from build123d import *

# Parameters (mm, degrees)
SKETCH1_R           = 0.8875
BOSS_EXTRUDE1_DEPTH = 2.5


with BuildPart() as part:
    # Sketch1 → Boss-Extrude1 (new body)
    with BuildSketch(Plane.XY):
        with BuildLine():
            Line((-40, 6.25), (-7.806247498, 6.25))
            ThreePointArc((-7.806247498, 6.25), (10, 0), (-7.806247498, -6.25))
            Line((-7.806247498, -6.25), (-40, -6.25))
            ThreePointArc((-40, -6.25), (-46.25, 0), (-40, 6.25))
        make_face()
        Circle(SKETCH1_R, mode=Mode.SUBTRACT)
        with Locations((-40, 0)):
            Circle(SKETCH1_R, mode=Mode.SUBTRACT)
        with Locations((0, 7.1)):
            Circle(SKETCH1_R, mode=Mode.SUBTRACT)
        with Locations((0, -7.1)):
            Circle(SKETCH1_R, mode=Mode.SUBTRACT)
        with Locations((-38.938319925, -3.387526445)):
            Circle(SKETCH1_R, mode=Mode.SUBTRACT)
        with BuildLine():
            ThreePointArc((-36.192394339, 2.278935142), (-38.420697766, 4.146951977), (-41.327100094, 4.234408057))
            ThreePointArc((-41.327100094, 4.234408057), (-41.908561687, 3.122106427), (-40.796260056, 2.540644834))
            ThreePointArc((-40.796260056, 2.540644834), (-39.05241866, 2.488171186), (-37.715436604, 1.367361085))
            ThreePointArc((-37.715436604, 1.367361085), (-36.498128443, 1.061626982), (-36.192394339, 2.278935142))
        make_face(mode=Mode.SUBTRACT)
        with BuildLine():
            ThreePointArc((-4.06945408, -1.769448993), (-1.980002796, -3.97127123), (1.035913802, -4.314891522))
            ThreePointArc((1.035913802, -4.314891522), (1.691709346, -3.244730457), (0.621548281, -2.588934913))
            ThreePointArc((0.621548281, -2.588934913), (-1.188001677, -2.382762738), (-2.441672448, -1.061669396))
            ThreePointArc((-2.441672448, -1.061669396), (-3.609453063, -0.601668379), (-4.06945408, -1.769448993))
        make_face(mode=Mode.SUBTRACT)
    extrude(amount=BOSS_EXTRUDE1_DEPTH)


solid = part.part
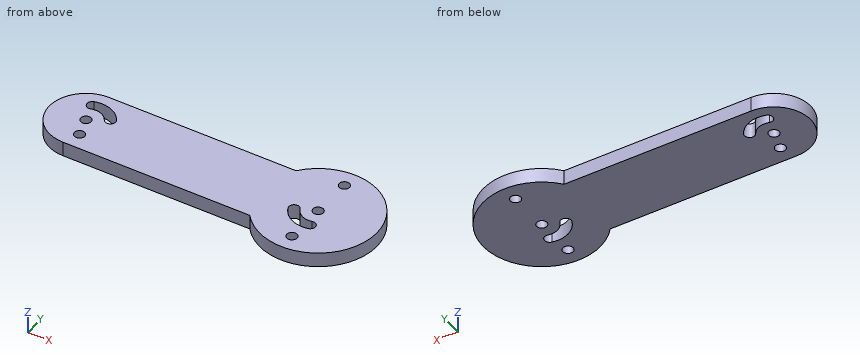
Model file for the job. Use its own axes, mm. Coordinates: 2 decimals unless noted, no trailing zeros. Order: outer loops, then holes, each group sorted by start corner. A loop starts at its lowest first (then second) coordinate and runs counter-clockwise, first axis right, second up. Notation, with made-up numbers: (26.25, 65) -> (48.25, 65) arc R35 cw to (48.25, 102) -> close; hole circle Ø10 at (26, 41.25). An arc over 180 degrees is marked (long way). Return JSON: item names as keys, results as strings. Group by question number.
Item 1: Saw through at D-D on y = 7.1. Write the cut outline in (x, z).
Item 2: Saw through at B-B on x = 0. Write the cut outline in (y, z).
Item 3: Saw through at C-C on z = 0.9. State how many separate pieces and enclosed holes the cut face has, then the cut area to 3 significant figures.
Item 4: Saw through at A-A on y = 0. Write the cut outline in (x, z).
Item 5: Flat gauge pins, fed straight in: P1, Ø10, axis at x = 4.5, y = 5, coming from the -Z side; P2, Ø0.8, axis at x = -31, z = 2, coming from the +Y side; P3, Ø1, axis at x = -15.5, z = 2, coming from the -Y side. Where does each tip first touch, or does it go through?
Item 6: Wall check: line 1 along Y through (x, z) = (0, 1.6); line 2 along X through (y, z) = (0.5, 0.6); line 3 along Y through (x, z) = (-25, 2.1). Give the ranges that are in metal, low to high. Write a range as [from, to].
Values found:
{
 "1": {"outline": "(-7.04, 0) -> (-0.89, 0) -> (-0.89, 2.5) -> (-7.04, 2.5) -> close; (0.89, 0) -> (7.04, 0) -> (7.04, 2.5) -> (0.89, 2.5) -> close"},
 "2": {"outline": "(-10, 0) -> (-7.99, 0) -> (-7.99, 2.5) -> (-10, 2.5) -> close; (-6.21, 0) -> (-4.44, 0) -> (-4.44, 2.5) -> (-6.21, 2.5) -> close; (-2.66, 0) -> (-0.89, 0) -> (-0.89, 2.5) -> (-2.66, 2.5) -> close; (0.89, 0) -> (6.21, 0) -> (6.21, 2.5) -> (0.89, 2.5) -> close; (7.99, 0) -> (10, 0) -> (10, 2.5) -> (7.99, 2.5) -> close"},
 "3": {"separate pieces": "1", "enclosed holes": "7", "area": "725 mm2"},
 "4": {"outline": "(-46.25, 0) -> (-40.89, 0) -> (-40.89, 2.5) -> (-46.25, 2.5) -> close; (-39.11, 0) -> (-0.89, 0) -> (-0.89, 2.5) -> (-39.11, 2.5) -> close; (0.89, 0) -> (10, 0) -> (10, 2.5) -> (0.89, 2.5) -> close"},
 "5": {"P1": "stops at z = 0", "P2": "stops at y = 6.25", "P3": "stops at y = -6.25"},
 "6": {"line 1": "y = [-10, -7.99], [-6.21, -4.44], [-2.66, -0.89], [0.89, 6.21], [7.99, 10]", "line 2": "x = [-46.23, -40.73], [-39.27, -0.73], [0.73, 9.99]", "line 3": "y = [-6.25, 6.25]"}
}
